from build123d import *

# Parameters (mm, degrees)
SKETCH_1_R      = 1.5
SKETCH_1_R_2    = 25
SKETCH_1_R_3    = 2
SKETCH_1_R_4    = 2.1
SKETCH_1_W      = 8.4
SKETCH_1_H      = 4.4
SKETCH_1_W_2    = 8.2
SKETCH_1_H_2    = 4.2
EXTRUDE_1_DEPTH = 4
FILLET_2_R      = 2


with BuildPart() as part:
    # 草图1 → 凸台-拉伸1 (new body)
    with BuildSketch(Plane.XY):
        with BuildLine():
            Line((7.027428163, -5.002489357), (20.810808237, -16.960441938))
            ThreePointArc((20.810808237, -16.960441938), (47.017847244, -26.746287876), (73.227648339, -16.967842153))
            Line((73.227648339, -16.967842153), (87.027428163, -5.002489357))
            Line((87.027428163, -5.002489357), (87.027428163, 75.054738201))
            Line((87.027428163, 75.054738201), (21.027428163, 141.054738201))
            Line((21.027428163, 141.054738201), (-114.887663771, 141.054738201))
            ThreePointArc((-114.887663771, 141.054738201), (-124.126459096, 134.881572525), (-121.958731583, 123.983670389))
            Line((-121.958731583, 123.983670389), (-90.203942848, 92.228881654))
            Line((-90.203942848, 92.228881654), (7.027428163, -5.002489357))
        make_face()
        with Locations((-52.972571837, 135.054738201)):
            Circle(SKETCH_1_R, mode=Mode.SUBTRACT)
        with Locations((47.027428163, 15.054738201)):
            Circle(SKETCH_1_R_2, mode=Mode.SUBTRACT)
        with Locations(Location((-22.972571837, 135.054738201, 0), (0, 0, 180))):
            Circle(SKETCH_1_R, mode=Mode.SUBTRACT)
        with Locations((7.027428163, 135.054738201)):
            Circle(SKETCH_1_R, mode=Mode.SUBTRACT)
        with Locations(Location((-112.972571837, 135.054738201, 0), (0, 0, 180))):
            Circle(SKETCH_1_R, mode=Mode.SUBTRACT)
        with Locations((-82.972571837, 135.054738201)):
            Circle(SKETCH_1_R, mode=Mode.SUBTRACT)
        with Locations((49.784787476, 103.812097514)):
            Circle(SKETCH_1_R, mode=Mode.SUBTRACT)
        with Locations(Location((70.997990912, 82.598894078, 0), (0, 0, 180))):
            Circle(SKETCH_1_R, mode=Mode.SUBTRACT)
        with Locations(Location((28.571584041, 125.025300949, 0), (0, 0, 180))):
            Circle(SKETCH_1_R, mode=Mode.SUBTRACT)
        with Locations((-83.04451802, 93.554738201)):
            Circle(SKETCH_1_R, mode=Mode.SUBTRACT)
        with Locations((-61.831314585, 72.341534765)):
            Circle(SKETCH_1_R, mode=Mode.SUBTRACT)
        with Locations(Location((-104.257721456, 114.767941637, 0), (0, 0, 180))):
            Circle(SKETCH_1_R, mode=Mode.SUBTRACT)
        with Locations((20.275835807, 57.054738201)):
            Circle(SKETCH_1_R, mode=Mode.SUBTRACT)
        with Locations((-6.58531727, 99.226748532)):
            Circle(SKETCH_1_R_3, mode=Mode.SUBTRACT)
        with Locations((70.527428163, -8.445261799)):
            Circle(SKETCH_1_R_4, mode=Mode.SUBTRACT)
        with Locations((23.527428163, -8.445261799)):
            Circle(SKETCH_1_R_4, mode=Mode.SUBTRACT)
        with Locations((23.527428163, 38.554738201)):
            Circle(SKETCH_1_R_4, mode=Mode.SUBTRACT)
        with Locations((70.527428163, 38.554738201)):
            Circle(SKETCH_1_R_4, mode=Mode.SUBTRACT)
        with Locations((-37.972571837, 135.054738201)):
            Rectangle(SKETCH_1_W, SKETCH_1_H, mode=Mode.SUBTRACT)
        with Locations((-7.972571837, 135.054738201)):
            Rectangle(SKETCH_1_W, SKETCH_1_H, mode=Mode.SUBTRACT)
        with Locations((-97.972571837, 135.054738201)):
            Rectangle(SKETCH_1_W, SKETCH_1_H, mode=Mode.SUBTRACT)
        with Locations((-67.972571837, 135.054738201)):
            Rectangle(SKETCH_1_W, SKETCH_1_H, mode=Mode.SUBTRACT)
        Polygon((55.865905794, 94.619709358), (61.805602756, 88.680012396), (64.916872594, 91.791282234), (58.977175632, 97.730979196), align=None, mode=Mode.SUBTRACT)
        Polygon((34.652702359, 115.832912794), (37.763972196, 118.944182631), (43.703669158, 113.004485669), (40.592399321, 109.893215832), align=None, mode=Mode.SUBTRACT)
        Polygon((-73.852129865, 87.473619883), (-76.963399702, 84.362350046), (-71.02370274, 78.422653084), (-67.912432903, 81.533922921), align=None, mode=Mode.SUBTRACT)
        Polygon((-89.125636339, 102.747126356), (-92.236906176, 99.635856519), (-98.176603138, 105.575553481), (-95.065333301, 108.686823318), align=None, mode=Mode.SUBTRACT)
        with Locations((5.275835807, 57.054738201)):
            Rectangle(SKETCH_1_W_2, SKETCH_1_H_2, mode=Mode.SUBTRACT)
        with Locations((35.275835807, 57.054738201)):
            Rectangle(SKETCH_1_W_2, SKETCH_1_H_2, mode=Mode.SUBTRACT)
        Polygon((-26.317798475, 106.3059132), (-58.783300448, 90.506724064), (-82.786741677, 114.510165293), (-76.96930946, 120.054738201), (-32.606331473, 120.054738201), align=None, mode=Mode.SUBTRACT)
        Polygon((47.299715686, 85.219705889), (24.926194473, 73.952189511), (4.862626833, 105.451990707), (-2.731253041, 122.054738201), (2.378929733, 122.054738201), align=None, mode=Mode.SUBTRACT)
        Polygon((-14.951358462, 60.079755544), (-17.922436994, 77.027703634), (-38.307901947, 67.107209668), (-24.754047946, 50.34609696), align=None, mode=Mode.SUBTRACT)
        Polygon((1.911503385, 33.57176286), (13.457428163, 19.475351063), (13.457428163, 30.764673398), align=None, mode=Mode.SUBTRACT)
    extrude(amount=EXTRUDE_1_DEPTH)

    # 圆角2
    fillet_2_edges = [part.edges().sort_by_distance(p)[0] for p in [
        (-26.317798475, 106.3059132, 2),
        (-32.606331473, 120.054738201, 2),
        (-76.96930946, 120.054738201, 2),
        (-82.786741677, 114.510165293, 2),
        (-58.783300448, 90.506724064, 2),
        (47.299715686, 85.219705889, 2),
        (2.378929733, 122.054738201, 2),
        (-2.731253041, 122.054738201, 2),
        (24.926194473, 73.952189511, 2),
        (-24.754047946, 50.34609696, 2),
        (-14.951358462, 60.079755544, 2),
        (-17.922436994, 77.027703634, 2),
        (-38.307901947, 67.107209668, 2),
        (13.457428163, 30.764673398, 2),
        (1.911503385, 33.57176286, 2),
        (13.457428163, 19.475351063, 2),
    ]]
    fillet(fillet_2_edges, radius=FILLET_2_R)


solid = part.part
Source: CAD feature listing. Evaluate the final solid. Frame: model axes, mm. A direction names the side the tool comes from. Coordinates: 2 decimals unless noted, no trailing zeros. Loops run counter-clockwise (first coordinate to the right, second up) from the corner with the lowest first, then second, coordinate; pieces in that order, holes last. Notation, with made-up numbers: M -32,16 L 17,16 A13 cw 17,38 Z; hole C 49,-22 d2. An arc over 180 degrees is marked long. Answer in a Markdown table with one row per item.
Q1. Set-up query: faces 1 (the flat face through (80.03, -11.07, 1.97)), 2 (the flat face through (-31.51, 58.7, 1.97)). Return all of +Z, -Z, +X, -X, +Y, -Y with unobstructed straight access to the full face (end or side cutting, diameter ignored); none if empty.
Answers below:
| item | result |
|---|---|
| face 1 | +Z, -Z, +X, -Y |
| face 2 | +Z, -Z |
Q2. Ray query, probe 1 along Y at (x, z) = (56.5, 1.35); probe 2 along X at (y, z) = (96.5, 2.5); probe 3 along Y at (x, z) = (-53, 3.2). Return the intervals inside material, ascending. Write a range as from..to.
Answers below:
| item | result |
|---|---|
| probe 1 | y = -25.61..-8.08, 38.19..93.99, 95.25..105.58 |
| probe 2 | x = -94.48..-64.78, -46.47..10.56, 33.54..57.75, 60.21..65.58 |
| probe 3 | y = 55.02..93.32, 120.05..133.55, 136.55..141.05 |
Q3. First-contact query: pin 1 (1.2 mm diameter, centred on y = 135, z = 2.5, fed in from +X); pin 2 (2 mm diameter, centred on x = -39.5, z = 2, fed in from -Y). Flat tips, straight axial feed; report the tip coordinate or a pass-through.
Answers below:
| item | result |
|---|---|
| pin 1 | stops at x = 27.68 |
| pin 2 | stops at y = 40.52 |
Q4. Section B-B on z = 0.75. State how many separate pieces and enclosed holes the cut face has, plus the area to 3 significant figures.
Answers below:
| item | result |
|---|---|
| separate pieces | 1 |
| enclosed holes | 32 |
| area | 16,400 mm^2 |
Q5. Draft query along Y for faces 3 (the flat face through (3, 77, 4)), 4 (the cylindrical face through (68.43, -8.35, 1.97)), 5 (the flat face through (-58.369, 60.393, 1.972)). Return one class per face: pulls with the +Y half, pulls with the -Y half, needs draft (parallel to the pull), parting line crosses it, or undercut.
Answers below:
| item | result |
|---|---|
| face 3 | needs draft |
| face 4 | undercut |
| face 5 | pulls with the -Y half |
Q6. Section A-A on y = 7.5. Return the cut outline in (x, z), plus the area to 3 significant figures.
Answers below:
| item | result |
|---|---|
| outline | M -5.48,0 L 23.2,0 L 23.2,4 L -5.48,4 Z; M 70.86,0 L 87.03,0 L 87.03,4 L 70.86,4 Z |
| area | 179 mm^2 |
